Model file for the job. Use its own axes, mm. Round coordinates to 2 decimals unless told otherwise and drop trailing zeros. Order: outer loops, then holes, each group sorted by start corner. A loop starts at its lowest first (then second) coordinate and runs counter-clockwise, first axis right, second up. Notation, with made-up numbers: (-26.5, 69) -> (-2.5, 69) arc R35 ccw to (-2.5, 101) -> close; hole circle Ø9 at (19, 30.5). An arc over 180 degrees is marked (long way). Use CSV: the item, a comma, the result in double quotes.
```python
from build123d import *

# Parameters (mm, degrees)
F1_DEPTH = 1.5875


with BuildPart() as f1:
    # F0 (on Top) → F1 (new body)
    with BuildSketch(Plane.XY):
        with BuildLine():
            ThreePointArc((10.583333, 0), (11.513269, 2.245064), (13.758333, 3.175))
            Line((13.758333, 3.175), (-14.816667, 4.7625))
            Line((-14.816667, 4.7625), (-24.341667, 0))
            Line((-24.341667, 0), (10.583333, 0))
        make_face()
        with BuildLine():
            ThreePointArc((13.758333, -3.175), (16.003397, -2.245064), (16.933333, 0))
            ThreePointArc((16.933333, 0), (16.003397, 2.245064), (13.758333, 3.175))
            ThreePointArc((13.758333, 3.175), (11.513269, 2.245064), (10.583333, 0))
            ThreePointArc((10.583333, 0), (11.513269, -2.245064), (13.758333, -3.175))
        make_face()
        with BuildLine():
            Line((-14.816667, -4.7625), (13.758333, -3.175))
            ThreePointArc((13.758333, -3.175), (11.513269, -2.245064), (10.583333, 0))
            Line((10.583333, 0), (-24.341667, 0))
            Line((-24.341667, 0), (-14.816667, -4.7625))
        make_face()
    extrude(amount=F1_DEPTH)


solid = f1.part
```
Q1. Cut at C-C (x = -17). Give the cut face in (y, z).
From the geometry:
outline,"(-3.67, 0) -> (3.67, 0) -> (3.67, 1.59) -> (-3.67, 1.59) -> close"
Q2. Probe line 1 along Y through (x, z) = (-21, 0.15); line 2 along X through (y, z) = (-1.25, 0.5); line 3 along Y through (x, z) = (15, 0.8). List the from-to ranges inside material, lowest first.
From the geometry:
line 1,"y = -1.67 to 1.67"
line 2,"x = -21.84 to 16.68"
line 3,"y = -2.92 to 2.92"
Q3. Cut at B-B (y = 1.5). Give the cut face in (x, z).
From the geometry:
outline,"(-21.34, 0) -> (16.56, 0) -> (16.56, 1.59) -> (-21.34, 1.59) -> close"
